Can you work these out from the model? Positions are in its coordinate system, mm. Face numbers are marked on the shaded views. Give positions to 0.01 mm unless a question says otherwise; leave off trailing zeros. Order: outer loops, then holes, each group sorted by start corner. A loop starts at its lowest first (then second) coordinate and runs counter-clockwise, first axis right, second up.
Item 1: If we mould it in two halves opening along Z, with no side actions, what happens to the marked faces 1, 2, 3 and 4? For each: +Z half, -Z half, draft (parallel to the pull), parting line (faces both ways), or undercut.
Item 2: I want a section at D-D, the plane x = 13. Write out the boundary of the cut face in (y, z).
Item 3: I want a section at A-A, the plane x = 36. Write out the boundary of the cut face in (y, z).
Item 4: If I drill on line 1 along Z through (x, y) = (37, 0.4); line 2 along X through (y, z) = (2.2, 1.4); line 3 along X through (y, z) = (-1.65, -0.45), over which ranges is the centre line in solid material (lowest first)?
Item 5: I want a section at B-B, the plane z = 0. Write out the boundary of the cut face in (x, y).
Item 6: I'm going to push flat-ended pins straight in: pin 1 Ø2 at (x, z) = (16.5, 1) entering from -Y; pin 2 Ø3 at (x, y) = (19, 1) entering from -Z. Where does each tip first touch, or does it pass through?
Item 7: I want a section at C-C, the plane y = 0. Write out the boundary of the cut face in (x, z).
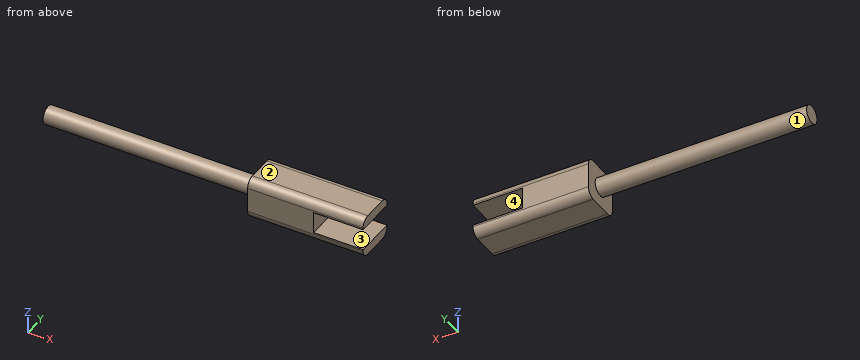
```python
from build123d import *

# Parameters (mm, degrees)
SKETCH1_R               = 1.09
BOSS_EXTRUDE1_DEPTH     = 27.637
BOSS_EXTRUDE2_DEPTH     = 14
CUT_EXTRUDE1_DEPTH      = 40.794368559
CUT_EXTRUDE1_DEPTH_BACK = 40.794368559
SKETCH3_W               = 7
SKETCH3_H               = 2.6


with BuildPart() as part:
    # Sketch1 → Boss-Extrude1 (new body)
    with BuildSketch(Plane(origin=(0, 0, 0), x_dir=(0, 0, -1), z_dir=(1, 0, 0))):
        with Locations(Location((0, 0, 0), (0, 0, 180))):
            Circle(SKETCH1_R)
    extrude(amount=BOSS_EXTRUDE1_DEPTH)

    # Sketch2 → Boss-Extrude2 (add)
    with BuildSketch(Plane(origin=(25.637, 0, 0), x_dir=(0, 0, -1), z_dir=(1, 0, 0))):
        with BuildLine():
            Line((-1.5, -2.5), (1.5, -2.5))
            ThreePointArc((1.5, -2.5), (2.207106781, -2.207106781), (2.5, -1.5))
            Line((2.5, -1.5), (2.5, 1.5))
            ThreePointArc((2.5, 1.5), (2.207106781, 2.207106781), (1.5, 2.5))
            Line((1.5, 2.5), (-1.5, 2.5))
            ThreePointArc((-1.5, 2.5), (-2.207106781, 2.207106781), (-2.5, 1.5))
            Line((-2.5, 1.5), (-2.5, -1.5))
            ThreePointArc((-2.5, -1.5), (-2.207106781, -2.207106781), (-1.5, -2.5))
        make_face()
    extrude(amount=BOSS_EXTRUDE2_DEPTH)

    # Sketch3 → Cut-Extrude1 (cut, two sides: drawn at the far end of the back side and taken through both)
    with BuildSketch(Plane(origin=(0, 0, 0), x_dir=(1, 0, 0), z_dir=(0, 1, 0)).offset(-CUT_EXTRUDE1_DEPTH_BACK)):
        with Locations((37.137, 0)):
            Rectangle(SKETCH3_W, SKETCH3_H)
    extrude(amount=CUT_EXTRUDE1_DEPTH + CUT_EXTRUDE1_DEPTH_BACK, mode=Mode.SUBTRACT)


solid = part.part
```
Results list:
1. face 1: parting line
1. face 2: +Z half
1. face 3: undercut
1. face 4: undercut
2. outline: circle Ø2.18 at (0, 0)
3. outline: (-2.5, -1.5) arc R1 ccw to (-1.5, -2.5) - (1.5, -2.5) arc R1 ccw to (2.5, -1.5) - (2.5, -1.3) - (-2.5, -1.3) - close; (-2.5, 1.3) - (2.5, 1.3) - (2.5, 1.5) arc R1 ccw to (1.5, 2.5) - (-1.5, 2.5) arc R1 ccw to (-2.5, 1.5) - close
4. line 1: z = -2.5 to -1.3, 1.3 to 2.5
4. line 2: x = 25.64 to 39.64
4. line 3: x = 25.64 to 33.64
5. outline: (0, -1.09) - (25.64, -1.09) - (25.64, -2.5) - (33.64, -2.5) - (33.64, 2.5) - (25.64, 2.5) - (25.64, 1.09) - (0, 1.09) - close
6. pin 1: stops at y = -1.09
6. pin 2: stops at z = -1.09
7. outline: (0, -1.09) - (25.64, -1.09) - (25.64, -2.5) - (39.64, -2.5) - (39.64, -1.3) - (33.64, -1.3) - (33.64, 1.3) - (39.64, 1.3) - (39.64, 2.5) - (25.64, 2.5) - (25.64, 1.09) - (0, 1.09) - close
